The model under review builds one solid part; all positions refer to its coordinate system, in mm. Face numbers are marked on the shaded views. Coordinates: 2 decimals unless noted, no trailing zeros. Order: outer loops, then holes, each group sorted by start corner. A loop starts at its lowest first (then second) coordinate and runs counter-clockwise, first axis right, second up. Notation, with made-up numbers: (-11.75, 11) -> (23.25, 11) arc R34 cw to (23.25, 42) -> close; hole circle Ø9 at (12, 18.25). An arc over 180 degrees is marked (long way). Use one line per item in the form item = value.
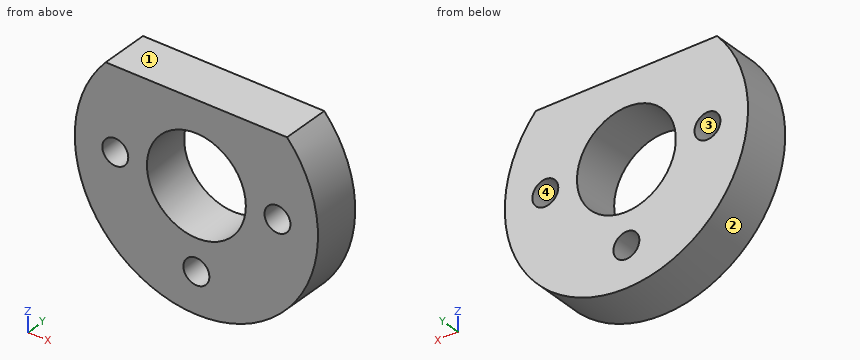
Autodesk Inventor part; units mm, degrees
ref_plane "YZ Plane" through (0, 0, 0) normal (1, 0, 0) x (0, 1, 0)
ref_plane "XZ Plane" through (0, 0, 0) normal (0, 1, 0) x (-1, 0, 0)
ref_plane "XY Plane" through (0, 0, 0) normal (0, 0, 1) x (1, 0, 0)
sketch "スケッチ1" plane through (0, 0, 0) normal (0, 1, 0) x (-1, 0, 0)
  circle A0 centre (0, 0) radius 15
  dimension "d0" = 30
extrude "押し出し1" add sketch "スケッチ1" along normal blind 6
sketch "スケッチ2" plane through (0, 6, 0) normal (0, 1, 0) x (1, 0, 0)
  arc A0 (2.6833, -3.1) -> (-2.6833, -3.1) centre (0, 0) ccw
  line L0 (-2.6833, -3.1) -> (2.6833, -3.1)
  point P0 (0, -3.1)
  dimension "d3" = 8.2
  dimension "d4" = 3.1
extrude "押し出し2" cut sketch "スケッチ2" against normal blind 6
sketch "スケッチ3" plane through (0, 6, 0) normal (0, 1, 0) x (1, 0, 0)
  circle A0 centre (0, 0) radius 15
  circle A1 centre (0, 0) radius 15
  line L0 (-11.1803, -10) -> (11.1803, -10)
  arc A2 (-11.1803, -10) -> (11.1803, -10) centre (0, 0) ccw
  point P0 (0, -10)
  dimension "d7" = 10
extrude "押し出し3" cut sketch "スケッチ3" against normal blind 6 contours L0 A0 picked at (2.8264, -10.7912)
sketch "スケッチ4" plane through (0, 6, 0) normal (0, 1, 0) x (1, 0, 0)
  circle A0 centre (0, 0) radius 10 construction
  point P0 (-10, 0)
  point P1 (0, 10)
  point P2 (10, 0)
  dimension "d10" = 20
hole "穴1" at (-10, 6, 0) at (0, 6, -10) at (10, 6, 0) direction (0, -1, 0) diameter 3.2 end through all
sketch "スケッチ5" plane through (0, 6, 0) normal (0, 1, 0) x (1, 0, 0)
  circle A0 centre (0, 0) radius 6.1
  dimension "d18" = 12.2
extrude "押し出し4" cut sketch "スケッチ5" against normal blind 10
properties part number "射出_留め具3"
Item 1: Draft analysis for pull direction X (two halves, no side actions). For the marked faces 1, 2, 3 and 4, state which applies: released by +X, released by -X, zero draft, split by the parting line, or undercut.
Results found:
face_1 = zero draft
face_2 = split by the parting line
face_3 = undercut
face_4 = undercut
Item 2: To check wall thickness, follow L1, parallel to Z at x = 0, y = 4.75; L2, parallel to Z at x = 10, y = 2.05; L3, parallel to X at y = 4.1, z = 0. State the ranges of each line that lie inside material, in increasing order. Write a range as from..to.
Results found:
L1 = -15..-11.6, -8.4..-6.1, 6.1..10
L2 = -11.18..-1.6, 1.6..10
L3 = -15..-11.6, -8.4..-6.1, 6.1..8.4, 11.6..15
Item 3: We need section C-C (z = -11.25). Write out the cut boundary in (x, y), plus the area to 3 significant figures.
Results found:
outline = (-9.92, 0) -> (-1, 0) -> (-1, 6) -> (-9.92, 6) -> close; (1, 0) -> (9.92, 0) -> (9.92, 6) -> (1, 6) -> close
area = 107 mm²
Item 4: We need section B-B (z = 0). Write out the cut boundary in (x, y).
Results found:
outline = (-15, 0) -> (-11.6, 0) -> (-11.6, 6) -> (-15, 6) -> close; (-8.4, 0) -> (-6.1, 0) -> (-6.1, 6) -> (-8.4, 6) -> close; (6.1, 0) -> (8.4, 0) -> (8.4, 6) -> (6.1, 6) -> close; (11.6, 0) -> (15, 0) -> (15, 6) -> (11.6, 6) -> close
Item 5: Clearance check with flat-ended pins moving along their axes: pin 1 (3 mm diameter, centred on y = 5, z = -10, fed in from +X); pin 2 (3.5 mm diameter, centred on x = 0, z = -10, fed in from +Y); pin 3 (3 mm diameter, centred on y = 2.5, z = -7.5, fed in from -X). State where each tip first meets the part, or that it passes through.
Results found:
pin_1 = 12.36
pin_2 = 6
pin_3 = -13.75
Item 6: We need section A-A (x = 0). Write out the cut boundary in (y, z), plus the area to 3 significant figures.
Results found:
outline = (0, -15) -> (6, -15) -> (6, -11.6) -> (0, -11.6) -> close; (0, -8.4) -> (6, -8.4) -> (6, -6.1) -> (0, -6.1) -> close; (0, 6.1) -> (6, 6.1) -> (6, 10) -> (0, 10) -> close
area = 57.6 mm²
Item 7: We need section D-D (y = 2). Write out the cut boundary in (x, z), plus the area to 3 significant figures.
Results found:
outline = (-11.18, 10) arc R15 ccw (long way) to (11.18, 10) -> close; hole circle Ø3.2 at (-10, 0); hole circle Ø12.2 at (0, 0); hole circle Ø3.2 at (0, -10); hole circle Ø3.2 at (10, 0)
area = 488 mm²
